Read the model definition and answer for the solid it produces. Units are mm, in the model's axes. Face numbers are marked on the shaded views. A direction names the side the tool comes from. Coordinates: 2 decimals unless noted, no trailing zeros. Order: outer loops, then holes, each group sorted by start corner. A loop starts at its lowest first (then second) coordinate and runs counter-clockwise, first axis right, second up.
from build123d import *

# Parameters (mm, degrees)
F0_W      = 125
F0_H      = 50
F1_DEPTH  = 50
F2_W      = 60
F2_H      = 25
F3_DEPTH  = 25
F4_R      = 17.5
F5_DEPTH  = 20
F6_R      = 5
F7_W      = 55
F7_H      = 10
F8_DEPTH  = 10
F9_R      = 3.5
F10_DEPTH = 25


with BuildPart() as f1:
    # F0 (on Front) → F1 (new body)
    with BuildSketch(Plane.XZ):
        with Locations((4.2377149548, 2.7714315802)):
            Rectangle(F0_W, F0_H)
    extrude(amount=F1_DEPTH)

    # F2 (on face) → F3 (cut)
    with BuildSketch(Plane.XZ.offset(50)):
        with Locations((36.7377149548, 15.2714315802)):
            Rectangle(F2_W, F2_H)
    extrude(amount=-F3_DEPTH, mode=Mode.SUBTRACT)

    # F4 (on face) → F5 (cut)
    with BuildSketch(Plane.XZ.offset(50)):
        with Locations((-25.7622850452, 2.7714315802)):
            Circle(F4_R)
    extrude(amount=-F5_DEPTH, mode=Mode.SUBTRACT)

    # F6
    f6_edges = [f1.edges().sort_by_distance(p)[0] for p in [
        (-25.762285, -50, 27.771432),
        (-58.262285, -50, 2.771432),
        (4.237715, -50, -22.228568),
        (66.737715, -50, -9.728568),
        (36.737715, -50, 2.771432),
        (6.737715, -50, 15.271432),
        (6.737715, -37.5, 27.771432),
        (36.737715, -25, 27.771432),
        (66.737715, -25, 15.271432),
        (66.737715, -37.5, 2.771432),
        (66.737715, -25, -22.228568),
        (66.737715, 0, 2.771432),
        (4.237715, 0, 27.771432),
        (4.237715, 0, -22.228568),
        (-58.262285, 0, 2.771432),
        (-58.262285, -25, 27.771432),
        (-58.262285, -25, -22.228568),
    ]]
    fillet(f6_edges, radius=F6_R)

    # F7 (on face) → F8 (cut)
    with BuildSketch(Plane.XY.offset(2.7714315802)):
        with Locations((34.2377149548, -35)):
            Rectangle(F7_W, F7_H)
    extrude(amount=-F8_DEPTH, mode=Mode.SUBTRACT)

    # F9 (on face) → F10 (cut)
    with BuildSketch(Plane.XY.offset(-7.2285684198)):
        with Locations((35.2377149548, -35.0629985332)):
            Circle(F9_R)
    extrude(amount=-F10_DEPTH, mode=Mode.SUBTRACT)


solid = f1.part
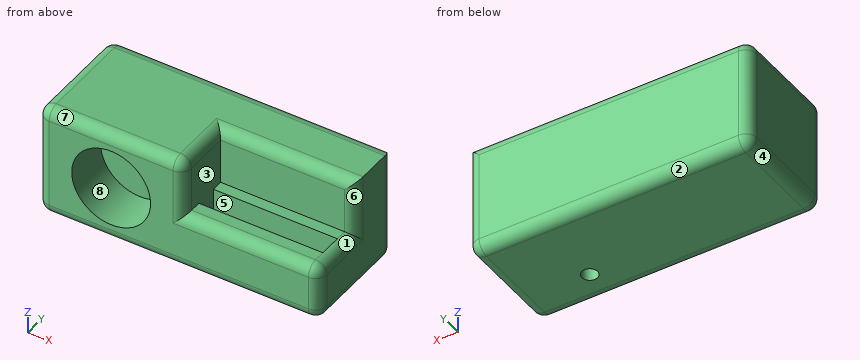
Q1. Which of the six approach directions +Z, -Z, +X, -X, +Y, -Y give full straight-line access (tool end or side, diameter ignored) to the marked faces 4, 5, 6, 7 and 8?
Q2. Determine the mould class of the marked faces 1, 2 and 3 for opening direction Y: +Y half, -Y half, draft (parallel to the pull), parting line (faces both ways), or undercut.
Q3. The part is cut by section B-B, the plane x = 55.5. Determine the outline of the cut face in (y, z).
Q4. The part is cut by section C-C, the plane z = -12. Determine the outline of the cut face in (x, y).
Q5. The part is cut by section D-D, the plane z = 18. Determine the outline of the cut face in (x, y).
Q6. The part is cut by section A-A, the plane y = -43.5. Determine the outline of the cut face in (x, z).
Q7. Straight lines are drawn through the part: L1, parallel to X at y = -30.5, z = -9; L2, parallel to Z at x = -25, y = -37; L3, parallel to Y at x = -38.5, z = -2. For each, find the intervals that lie inside material, in ascending order.
Q8. Each of these flat-tipped pins is pushed along its axis until it touches: P1, Ø2, axis at y = -45, z = 21, coming from the +X side; P2, Ø5, axis at x = 42.5, y = -34, coming from the +Z side; P3, Ø2.5, axis at x = 42.5, y = -43, coming from the +Z side. Where does it stop, or does it pass through?
Computed values:
1. face 4: -Z, -X, +Y, -Y
1. face 5: +Z
1. face 6: +Z, +X, -Y
1. face 7: +Z, +X, -X, -Y
1. face 8: -Y
2. face 1: draft
2. face 2: +Y half
2. face 3: undercut
3. outline: (-50, -17.23) arc R5 ccw to (-45, -22.23) - (-5, -22.23) arc R5 ccw to (0, -17.23) - (0, 22.77) arc R5 ccw to (-5, 27.77) - (-20, 27.77) arc R5 ccw to (-25, 22.77) - (-25, 2.77) - (-30, 2.77) - (-30, -7.23) - (-40, -7.23) - (-40, 2.77) - (-45, 2.77) arc R5 ccw to (-50, -2.23) - close
4. outline: (-58.26, -45) arc R5 ccw to (-53.26, -50) - (-35.15, -50) - (-35.15, -30) - (-16.38, -30) - (-16.38, -50) - (61.74, -50) arc R5 ccw to (66.74, -45) - (66.74, -5) arc R5 ccw to (61.74, 0) - (-53.26, 0) arc R5 ccw to (-58.26, -5) - close; hole circle Ø7 at (35.24, -35.06)
5. outline: (-58.26, -45) arc R5 ccw to (-53.26, -50) - (-34.38, -50) - (-34.38, -30) - (-17.14, -30) - (-17.14, -50) - (1.74, -50) arc R5 ccw to (6.74, -45) - (6.74, -25) - (61.74, -25) arc R5 ccw to (66.74, -20) - (66.74, -5) arc R5 ccw to (61.74, 0) - (-53.26, 0) arc R5 ccw to (-58.26, -5) - close
6. outline: (-58.26, -17.23) arc R5 ccw to (-53.26, -22.23) - (61.74, -22.23) arc R5 ccw to (66.74, -17.23) - (66.74, -2.23) arc R5 ccw to (61.74, 2.77) - (6.74, 2.77) - (6.74, 22.77) arc R5 ccw to (1.74, 27.77) - (-53.26, 27.77) arc R5 ccw to (-58.26, 22.77) - close; hole circle Ø35 at (-25.76, 2.77)
7. L1: x = -58.26 to -38.71, -12.81 to 66.74
7. L2: z = -22.23 to -14.71, 20.25 to 27.77
7. L3: y = -30 to 0
8. P1: stops at x = 6.74
8. P2: stops at z = -7.23
8. P3: stops at z = 2.77
